The model under review builds one solid part; all positions refer to its coordinate system, in mm. A direction names the side the tool comes from. Coordinates: 2 decimals unless noted, no trailing zeros. Order: outer loops, then holes, each group sorted by start corner. A loop starts at its lowest first (then second) coordinate and runs counter-clockwise, first axis right, second up. Notation, with made-up numbers: M 82.25,67 L 128.25,67 A20 cw 128.25,86 Z; hole C 46,44 d10. An arc over 180 degrees is marked long. Write each question's results on one line, items separated by ' | '.
Autodesk Inventor part; units mm, degrees
ref_plane "YZ Plane" through (0, 0, 0) normal (1, 0, 0) x (0, 1, 0)
ref_plane "XZ Plane" through (0, 0, 0) normal (0, 1, 0) x (-1, 0, 0)
ref_plane "XY Plane" through (0, 0, 0) normal (0, 0, 1) x (1, 0, 0)
sketch "Sketch1" plane through (0, 0, 0) normal (0, 1, 0) x (-1, 0, 0)
  line L0 (-17.5, 27.5) -> (17.5, 27.5)
  line L1 (-17.5, 27.5) -> (17.5, -27.5) construction
  line L2 (17.5, 27.5) -> (-17.5, -27.5) construction
  circle A0 centre (10.5, 4.5) radius 5.5
  circle A1 centre (-10.5, 4.5) radius 5.5
  circle A2 centre (-10.5, 20.5) radius 5.5
  circle A3 centre (10.5, 20.5) radius 5.5
  line L3 (17.5, 27.5) -> (17.5, -16.5)
  line L4 (-17.5, 27.5) -> (-17.5, -16.5)
  circle A4 centre (0, -16.5) radius 8
  line L5 (8, -27.5) -> (-8, -27.5)
  arc A5 (8, -27.5) -> (17.5, -16.5) centre (7.5511, -17.5101) ccw
  arc A6 (-17.5, -16.5) -> (-8, -27.5) centre (-7.5511, -17.5101) ccw
  point P0 (0, 0)
  point P1 (0, 27.5)
  dimension "d0" = 35
  dimension "d1" = 55
  dimension "d5" = 11
  dimension "d7" = 11
  dimension "d9" = 11
  dimension "d11" = 11
  dimension "d13" = 7
  dimension "d15" = 23
  dimension "d16" = 21
  dimension "d17" = 10.5
  dimension "d18" = 44
  dimension "d19" = 16
  dimension "d20" = 44
  dimension "d25" = 10
  dimension "d26" = 10
extrude "Extrusion1" add sketch "Sketch1" along normal blind 7
sketch "Sketch2" plane through (0, 7, 0) normal (0, 1, 0) x (1, 0, 0)
  line L0 (-17.5, 16.5) -> (-17.5, -27.5)
  line L1 (-17.5, -27.5) -> (-17.5, 16.5)
  line L2 (8, 27.5) -> (-8, 27.5)
  line L3 (-8, 27.5) -> (8, 27.5)
  line L4 (17.5, -27.5) -> (17.5, 16.5)
  line L5 (17.5, 16.5) -> (17.5, -27.5)
  line L6 (-17.5, -27.5) -> (17.5, -27.5)
  line L7 (17.5, -27.5) -> (-17.5, -27.5)
  circle A0 centre (0, 16.5) radius 8
  circle A1 centre (-10.5, -4.5) radius 3
  circle A2 centre (10.5, -4.5) radius 3
  circle A3 centre (10.5, -20.5) radius 3
  circle A4 centre (-10.5, -20.5) radius 3
  arc A5 (-8, 27.5) -> (-17.5, 16.5) centre (-7.5511, 17.5101) ccw
  arc A6 (-8, 27.5) -> (-17.5, 16.5) centre (-7.5511, 17.5101) ccw
  arc A7 (17.5, 16.5) -> (8, 27.5) centre (7.5511, 17.5101) ccw
  point P0 (0, 0)
  point P1 (0, -27.5)
  dimension "d29" = 16
  dimension "d30" = 6
  dimension "d31" = 6
  dimension "d32" = 6
  dimension "d33" = 6
  dimension "d34" = 7
  dimension "d35" = 23
  dimension "d36" = 21
  dimension "d37" = 10.5
extrude "Extrusion2" add sketch "Sketch2" along normal blind 13
properties part number "spindel sockel" material "Steel"
1) To check wall thickness, follow line 1 along Z through (x, y) = (-10.5, 16.75); line 2 along Z through (x, y) = (10.5, 3.75); line 3 along X through (y, z) = (3.25, 0). State the ranges of each line that lie inside material, in increasing order.
Solutions:
line 1: -27.07 to 1.5, 7.5 to 17.5, 23.5 to 27.5 | line 2: -27.07 to -1, 10 to 15, 26 to 27.5 | line 3: -17.5 to -13.66, -7.34 to 7.34, 13.66 to 17.5
2) Take a section at A-A on y = 4.5. State the section outline as (x, z) points.
Solutions:
outline: M -17.5,-16.5 A10 ccw -8,-27.5 L 8,-27.5 A10 ccw 17.5,-16.5 L 17.5,27.5 L -17.5,27.5 Z; hole C -10.5,4.5 d11; hole C -10.5,20.5 d11; hole C 0,-16.5 d16; hole C 10.5,4.5 d11; hole C 10.5,20.5 d11
3) For pin 1 (6 mm diameter, centred on x = -13, y = 6, fed in from -Z); pin 2 (5 mm diameter, centred on y = 12, z = 19.5, fed in from -X); pin 3 (9.5 mm diameter, centred on x = 10.5, z = 20.5, fed in from -Y), all flat-tipped, find the tip position at first contact; note any pin that passes through.
Solutions:
pin 1: z = -27.21 | pin 2: x = -17.5 | pin 3: y = 7
4) Take a section at C-C on x = 10.5. State the section outline as (y, z) points.
Solutions:
outline: M 0,-27.07 L 20,-27.07 L 20,1.5 L 7,1.5 L 7,-1 L 0,-1 Z; M 0,10 L 7,10 L 7,7.5 L 20,7.5 L 20,17.5 L 7,17.5 L 7,15 L 0,15 Z; M 0,26 L 7,26 L 7,23.5 L 20,23.5 L 20,27.5 L 0,27.5 Z
5) The part is to be moulded in two halves that separate along X. For faces 4 (the cylindrical face through (15.044, 9.86, -24.132)), 5 (the flat face through (0, 20, 0)), 6 (the flat face through (-8, 7, 7)), 7 (the cylindrical face through (-12.9, 13.4, 18.7)), say which applies: pulls with the +X half, pulls with the -X half, needs draft (parallel to the pull), parting line crosses it, or undercut.
Solutions:
face 4: pulls with the +X half | face 5: needs draft | face 6: undercut | face 7: undercut
6) Take a section at B-B on z = 4.5. State the section outline as (x, y) points, plus the area to 3 significant figures.
Solutions:
outline: M -17.5,0 L -16,0 L -16,7 L -13.5,7 L -13.5,20 L -17.5,20 Z; M -7.5,7 L -5,7 L -5,0 L 5,0 L 5,7 L 7.5,7 L 7.5,20 L -7.5,20 Z; M 13.5,7 L 16,7 L 16,0 L 17.5,0 L 17.5,20 L 13.5,20 Z | area: 390 mm2
7) Take a section at D-D on z = -17.5. State the section outline as (x, y) points, plus the area to 3 significant figures.
Solutions:
outline: M -17.55,0 L -7.94,0 L -7.94,20 L -17.55,20 Z; M 7.94,0 L 17.55,0 L 17.55,20 L 7.94,20 Z | area: 385 mm2
8) For faces 1 (the cylindrical face through (0.527, 9.86, -8.517)), 2 (the cylindrical face through (5.42, 3.45, 6.61)), 3 (the flat face through (17.5, 10, 6)), list the 3-axis set-ups (+Z, -Z, +X, -X, +Y, -Y) from which the entire face can be reached by the end or side of a thin tool; tool diameter is ignored.
Solutions:
face 1: +Y, -Y | face 2: -Y | face 3: +Z, +X, +Y, -Y
